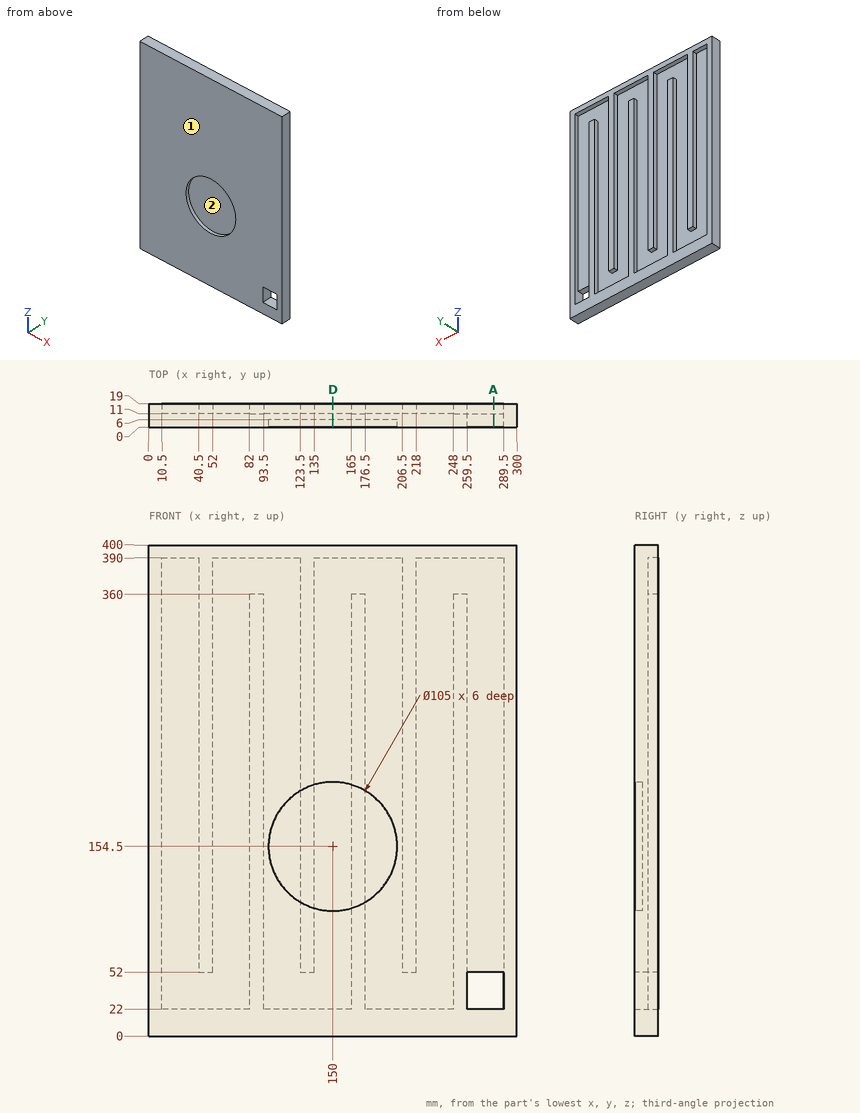
Input: dimensioned drawing with shaded views. Units: mm. Origin: part minimum x, y, z. Round coordinates to 2 decimals unless told otherwise and drop trailing zeros. Loops run counter-clockwise (first coordinate to the right, second up) from the corner with the lowest first, then second, coordinate; pieces in that order, holes last. Notation, with made-up numbers: (75.5, 63.5) -> (106.5, 63.5) arc R32 ccw to (106.5, 99.5) -> close; hole circle Ø3 at (75, 88). An arc over 180 degrees is marked (long way). Answer as a JSON object with one key per item and string values. Group by question number.
1) Ray query, L1, parallel to X at y = 12, z = 49; L2, parallel to Z at x = 213, y = 17.5; L3, parallel to Z at x = 150, y = 2.55. Return the intervals inside material, ascending.
2) Section query D-D on x = 150. Output: boundary loops of the cut face in (y, z).
3) Pin query (flat end, axial travel): pin 1 (4 mm diameter, centred on y = 16.5, z = 299, fed in from -X); pin 2 (3 mm diameter, centred on x = 113.5, z = 135, fed in from +Y). Return the tip coordinate at first contact, or that it passes through.
4) Section query A-A on x = 281. Output: boundary loops of the cut face in (y, z).
5) Draft query along Z for the marked faces 1 and 2. Return one class per face: +Z half, -Z half, draft (parallel to the pull), parting line (faces both ways), or undercut.
Reply:
{
 "1": {"L1": "x = 0 to 10.5, 82 to 93.5, 165 to 176.5, 248 to 259.5, 289.5 to 300", "L2": "z = 0 to 22, 52 to 400", "L3": "z = 0 to 102, 207 to 400"},
 "2": {"outline": "(0, 0) -> (19, 0) -> (19, 22) -> (11, 22) -> (11, 390) -> (19, 390) -> (19, 400) -> (0, 400) -> (0, 207) -> (6, 207) -> (6, 102) -> (0, 102) -> close"},
 "3": {"pin 1": "stops at x = 0", "pin 2": "stops at y = 11"},
 "4": {"outline": "(0, 0) -> (19, 0) -> (19, 22) -> (0, 22) -> close; (0, 52) -> (11, 52) -> (11, 390) -> (19, 390) -> (19, 400) -> (0, 400) -> close"},
 "5": {"face 1": "draft", "face 2": "undercut"}
}
